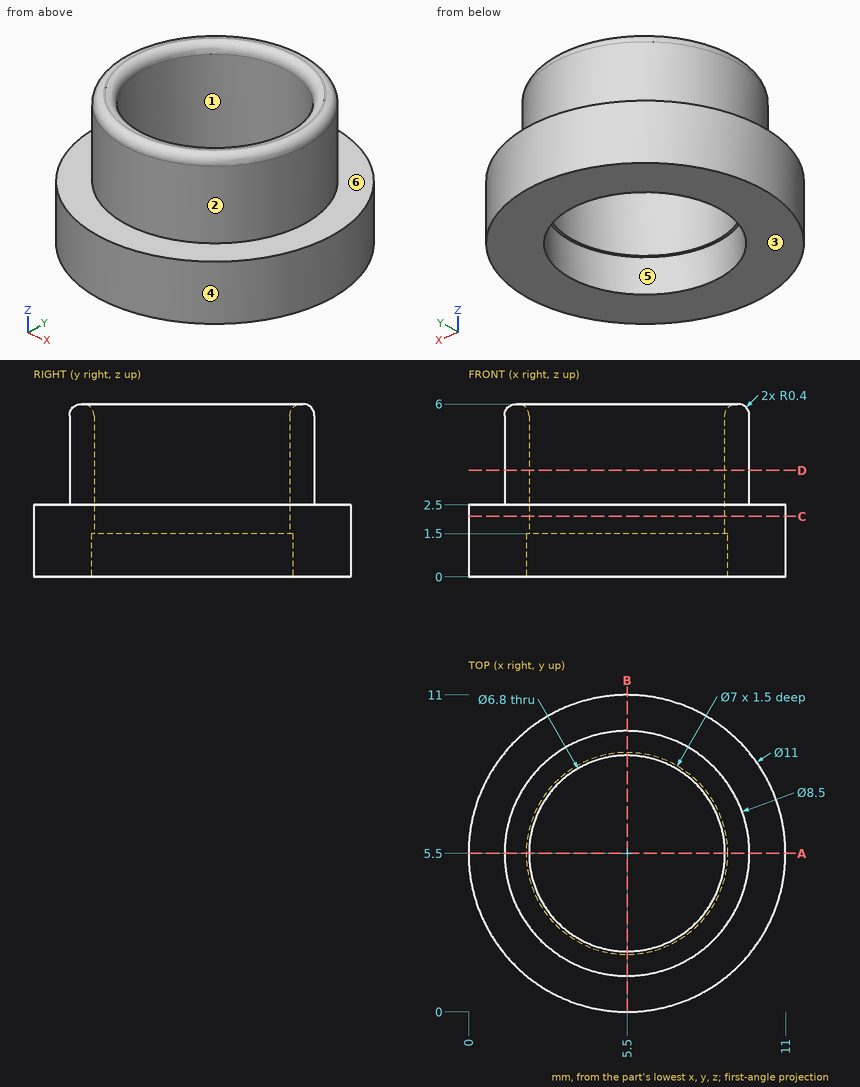
Source: three-view drawing plus pictorial views. Frame: mm from the lowest corner of the part. A direction names the side the tool comes from. Give positions to 0.01 mm unless a question says otherwise; leave off trailing zeros. Order: outer loops, then holes, each group sorted by start corner. A loop starts at its lowest first (then second) coordinate and runs counter-clockwise, first axis right, second up. Notation, with made-up numbers: M 64.5,16 L 71.5,16 A31 ccw 71.5,49 Z; hole C 46.5,46.25 d2. An arc over 180 degrees is marked long. One line per question, with ' | ' between items. Start each with the question number.
1. Access query for the marked faces 4, 5 and 6. Directions: +Z, -Z, +X, -X, +Y, -Y. A direction counts if a zero-diameter tool reaches every point of the face in a straight line with its end or side. Return the directions, or none.
2. Section query C-C (z = 2.1). Return the cut outline in (x, y), and give its area (3 significant figures).
3. Section query A-A (y = 5.5). Return the cut outline in (x, z).
4. Pull-direction query (Y, two-part tool) for the marked faces 1, 2 and 3; classes: released by +Y, released by -Y, zero draft, split by the parting line, or undercut.
5. Material intervals for probe 1 along Y at (x, z) = (5.5, 1.15); probe 2 along Z at (x, y) = (9.75, 2.5); probe 3 along Y at (x, z) = (8, 1.7), sorted ascending. Write a range as [from, to].
6. First-contact query: pin 1 Ø6.5 at (x, y) = (5.5, 5.5) entering from -Z; pin 2 Ø2 at (y, z) = (2.5, 2.5) entering from -X; pin 3 Ø3 at (y, z) = (3, 1.5) entering from +X; pin 4 Ø1.5 at (x, z) = (3, 3) entering from +Y. Flat tips, straight axial feed; report the tip coordinate or a pass-through.
7. Section query D-D (z = 3.7). Return the cut outline in (x, y).
Here are the results:
1) face 4: +Z, -Z | face 5: -Z | face 6: +Z
2) outline: C 5.5,5.5 d11; hole C 5.5,5.5 d6.8 | area: 58.7 mm²
3) outline: M 0,0 L 2,0 L 2,1.5 L 2.1,1.5 L 2.1,5.6 A0.4 ccw 1.7,6 L 1.65,6 A0.4 ccw 1.25,5.6 L 1.25,2.5 L 0,2.5 Z; M 8.9,1.5 L 9,1.5 L 9,0 L 11,0 L 11,2.5 L 9.75,2.5 L 9.75,5.6 A0.4 ccw 9.35,6 L 9.3,6 A0.4 ccw 8.9,5.6 Z
4) face 1: undercut | face 2: split by the parting line | face 3: zero draft
5) probe 1: [0, 2], [9, 11] | probe 2: [0, 2.5] | probe 3: [0.6, 3.2], [7.8, 10.4]
6) pin 1: through | pin 2: x = 0.38 | pin 3: x = 10.91 | pin 4: y = 10.65
7) outline: C 5.5,5.5 d8.5; hole C 5.5,5.5 d6.8
